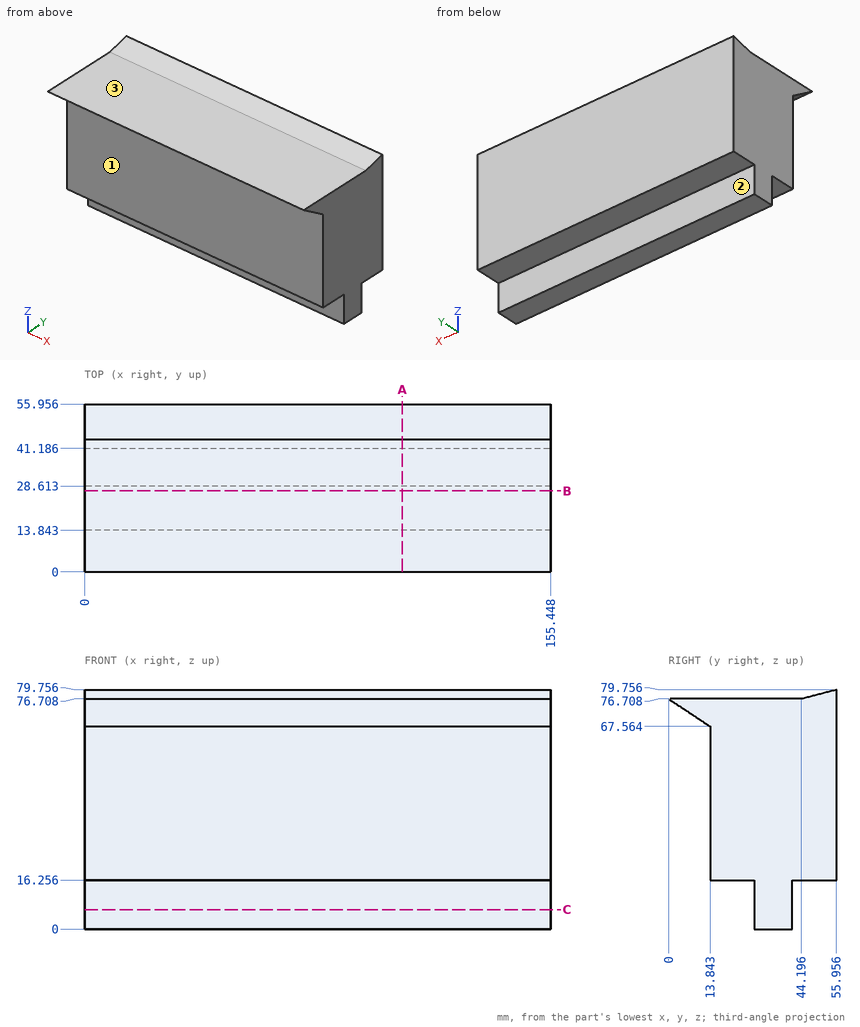
Geometry: see drawing. Coordinates: mm, zero at the bounding-box minimum. A direction names the side the tool comes from. Round coordinates to 2 decimals unless told otherwise and drop trailing zeros. Write each loop counter-clockwise with the first axis right and the second up, starting at its lowest first coordinate (ties: lowest second). Pieces come first, ordered by that corner, then holes.
1) Ray query, L1, parallel to Y at x = 28.5, z = 6.5; L2, parallel to Y at x = 96.5, z = 30.5; L3, parallel to Z at x = 67.5, y = 15. Return the intervals inside material, ascending.
2) Reachability of the marked faces 1, 2 and 3 from +Z, -Z, +X, -X, +Y, -Y: full face, straight path, thin tool, end or side. Return the list, or none.
3) Cut plane B-B (y = 27). Return the cut outline in (x, z).
4) Cut plane C-C (z = 6.5). Return the cut outline in (x, y).
5) Contact query for flat-ended pins moving along their axis: P1, Ø4.5, axis at x = 54, y = 49, coming from the -Z side; P2, Ø18, axis at x = 77.5, z = 5, coming from the -Y side; P3, Ø22, axis at x = 40, y = 19.5, coming from the +Z side. Output: stop coordinate, or through.
6) Cut plane A-A (x = 106). Return the cut outline in (y, z), then the cut area to 3 significant figures.
Geometry says:
1. L1: y = 28.61 to 41.19
1. L2: y = 13.84 to 55.96
1. L3: z = 16.26 to 76.71
2. face 1: -Z, +X, -X, -Y
2. face 2: -Z, +X, -X, +Y
2. face 3: +Z, +X, -X, -Y
3. outline: (0, 16.26) - (155.45, 16.26) - (155.45, 76.71) - (0, 76.71) - close
4. outline: (0, 28.61) - (155.45, 28.61) - (155.45, 41.19) - (0, 41.19) - close
5. P1: stops at z = 16.26
5. P2: stops at y = 28.61
5. P3: stops at z = 76.71
6. outline: (0, 76.71) - (13.84, 67.56) - (13.84, 16.26) - (28.61, 16.26) - (28.61, 0) - (41.19, 0) - (41.19, 16.26) - (55.96, 16.26) - (55.96, 79.76) - (44.2, 76.71) - close
6. area: 2,830 mm2
